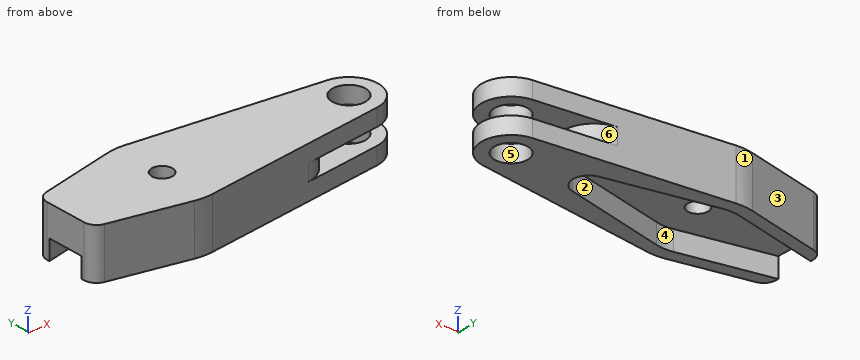
```python
from build123d import *

# Parameters (mm, degrees)
SKETCH2_R               = 2.625
BOSS_EXTRUDE2_DEPTH     = 8
CUT_EXTRUDE5_DEPTH      = 3.15
CUT_EXTRUDE6_DEPTH      = 37.482230264
CUT_EXTRUDE6_DEPTH_BACK = 37.482230264
SKETCH6_W               = 24
SKETCH6_H               = 2.6
FILLET1_R               = 5
CUT_EXTRUDE7_DEPTH      = 37.482230264
CUT_EXTRUDE7_DEPTH_BACK = 37.482230264
SKETCH1_7_R             = 1.625
SKETCH7_W               = 26.970959806
SKETCH7_H               = 23.004642188
CUT_EXTRUDE8_DEPTH      = 37.482230264
FILLET2_R               = 2


with BuildPart() as part:
    # Sketch2 → Boss-Extrude2 (new body)
    with BuildSketch(Plane.XY):
        with BuildLine():
            Line((-1.767857143, 8.058360945), (-18.464285714, 4.395469606))
            ThreePointArc((-18.464285714, 4.395469606), (-22, 0), (-18.464285714, -4.395469606))
            Line((-18.464285714, -4.395469606), (-1.767857143, -8.058360945))
            ThreePointArc((-1.767857143, -8.058360945), (-0.391032035, -8.240727756), (0.996875, -8.189550674))
            Line((0.996875, -8.189550674), (30.558854167, -4.591111741))
            ThreePointArc((30.558854167, -4.591111741), (34.625, 0), (30.558854167, 4.591111741))
            Line((30.558854167, 4.591111741), (0.996875, 8.189550674))
            ThreePointArc((0.996875, 8.189550674), (-0.391032035, 8.240727756), (-1.767857143, 8.058360945))
        make_face()
        with Locations((30, 0)):
            Circle(SKETCH2_R, mode=Mode.SUBTRACT)
    extrude(amount=BOSS_EXTRUDE2_DEPTH)

    # Sketch1 → Cut-Extrude5 (cut)
    with BuildSketch(Plane.XY):
        with BuildLine():
            Line((-1.339285714, 6.104818898), (-18.035714286, 2.441927559))
            ThreePointArc((-18.035714286, 2.441927559), (-20, 0), (-18.035714286, -2.441927559))
            Line((-18.035714286, -2.441927559), (-1.339285714, -6.104818898))
            ThreePointArc((-1.339285714, -6.104818898), (0, -6.25), (1.339285714, -6.104818898))
            Line((1.339285714, -6.104818898), (18.035714286, -2.441927559))
            ThreePointArc((18.035714286, -2.441927559), (20, 0), (18.035714286, 2.441927559))
            Line((18.035714286, 2.441927559), (1.339285714, 6.104818898))
            ThreePointArc((1.339285714, 6.104818898), (0, 6.25), (-1.339285714, 6.104818898))
        make_face()
    extrude(amount=CUT_EXTRUDE5_DEPTH, mode=Mode.SUBTRACT)

    # Sketch6 → Cut-Extrude6 (cut, two sides: drawn at the far end of the back side and taken through both)
    with BuildSketch(Plane(origin=(0, 0, 0), x_dir=(1, 0, 0), z_dir=(0, 1, 0)).offset(-CUT_EXTRUDE6_DEPTH_BACK)):
        with Locations((34.625, -4)):
            Rectangle(SKETCH6_W, SKETCH6_H)
    extrude(amount=CUT_EXTRUDE6_DEPTH + CUT_EXTRUDE6_DEPTH_BACK, mode=Mode.SUBTRACT)

    # Fillet1
    fillet1_edges = [part.edges().sort_by_distance(p)[0] for p in [
        (22.625, 5.556862023, 4),
        (22.625, -5.556862023, 4),
    ]]
    fillet(fillet1_edges, radius=FILLET1_R)

    # Sketch1<7> → Cut-Extrude7 (cut, two sides: drawn at the far end of the back side and taken through both)
    with BuildSketch(Plane.XY.offset(-CUT_EXTRUDE7_DEPTH_BACK)):
        Circle(SKETCH1_7_R)
    extrude(amount=CUT_EXTRUDE7_DEPTH + CUT_EXTRUDE7_DEPTH_BACK, mode=Mode.SUBTRACT)

    # Sketch7 → Cut-Extrude8 (cut, through all)
    with BuildSketch(Plane.XY):
        with Locations((-28.985479903, 0)):
            Rectangle(SKETCH7_W, SKETCH7_H)
    extrude(amount=CUT_EXTRUDE8_DEPTH, mode=Mode.SUBTRACT)

    # Fillet2
    fillet2_edges = [part.edges().sort_by_distance(p)[0] for p in [
        (-15.5, -5.045779726, 4),
        (-15.5, 5.045779726, 4),
    ]]
    fillet(fillet2_edges, radius=FILLET2_R)


solid = part.part
```
Input: part model. Units: mm. Frame: model coordinates. Face numbers are marked on the shaded views. A direction names the side the tool comes from. Round coordinates to 2 decimals unless told otherwise and drop trailing zeros. Loops run counter-clockwise (first coordinate to the right, second up) from the corner with the lowest first, then second, coordinate; pieces in that order, holes last.
1) Section query D-D on x = 30. Return the cut outline in (y, z) (3 decimals).
Ans:
outline: (-4.659, 0) - (-2.625, 0) - (-2.625, 2.7) - (-4.659, 2.7) - close; (-4.659, 5.3) - (-2.625, 5.3) - (-2.625, 8) - (-4.659, 8) - close; (2.625, 0) - (4.659, 0) - (4.659, 2.7) - (2.625, 2.7) - close; (2.625, 5.3) - (4.659, 5.3) - (4.659, 8) - (2.625, 8) - close
2) Section query A-A on x = 0. Return the cut outline in (y, z) (3 decimals).
Ans:
outline: (-8.25, 0) - (-6.25, 0) - (-6.25, 3.15) - (-1.625, 3.15) - (-1.625, 8) - (-8.25, 8) - close; (1.625, 3.15) - (6.25, 3.15) - (6.25, 0) - (8.25, 0) - (8.25, 8) - (1.625, 8) - close
3) Material intervals for line 1 (X direction, y = 0, z = 7.35) (3 decimals); line 2 (Y direction, x = 0, z = 4.25) (3 decimals); line 3 (Z direction, x = 26, y = -3.5), sorted ascending.
Ans:
line 1: x = -15.5 to -1.625, 1.625 to 27.375, 32.625 to 34.625
line 2: y = -8.25 to -1.625, 1.625 to 8.25
line 3: z = 0 to 2.7, 5.3 to 8
4) Section query C-C on y = 0. Return the cut outline in (x, z) (3 decimals).
Ans:
outline: (-15.5, 3.15) - (-1.625, 3.15) - (-1.625, 8) - (-15.5, 8) - close; (1.625, 3.15) - (20, 3.15) - (20, 0) - (27.375, 0) - (27.375, 2.7) - (22.625, 2.7) - (22.625, 5.3) - (27.375, 5.3) - (27.375, 8) - (1.625, 8) - close; (32.625, 0) - (34.625, 0) - (34.625, 2.7) - (32.625, 2.7) - close; (32.625, 5.3) - (34.625, 5.3) - (34.625, 8) - (32.625, 8) - close
5) Set-up query: the marked faces 4, 5 and 6. Return all of +Z, -Z, +X, -X, +Y, -Y with unobstructed straight access to the full face (end or side cutting, diameter ignored); none if empty.
Ans:
face 4: -Z
face 5: +Z, -Z
face 6: +X, +Y
6) Pin query (flat end, axial travel): pin 1 (2.5 mm diameter, centred on y = -0.5, z = 4, fed in from +X) (3 decimals); pin 2 (3 mm diameter, centred on x = 9.5, y = -1.5, fed in from -Z); pin 3 (1.5 mm diameter, centred on x = -4.5, z = 2.5, fed in from +Y). Return the tip coordinate at first contact, or that it passes through.
Ans:
pin 1: stops at x = 22.625
pin 2: stops at z = 3.15
pin 3: stops at y = 7.62
7) Section query B-B on z = 5.75. Return the cut outline in (x, y) (3 decimals), plus the area to 3 significant figures.
Ans:
outline: (-15.5, -3.437) arc R2 ccw to (-13.929, -5.391) - (-1.768, -8.058) arc R8.25 ccw to (0.997, -8.19) - (30.559, -4.591) arc R4.625 ccw to (30.559, 4.591) - (0.997, 8.19) arc R8.25 ccw to (-1.768, 8.058) - (-13.929, 5.391) arc R2 ccw to (-15.5, 3.437) - close; hole circle Ø3.25 at (0, 0); hole circle Ø5.25 at (30, 0)
area: 601 mm2
8) Pull-direction query (X, two-part tool) for the marked faces 1, 2 and 3; classes: released by +X, released by -X, zero draft, split by the parting line, or undercut.
Ans:
face 1: split by the parting line
face 2: undercut
face 3: released by -X
